```python
from build123d import *

# Parameters (mm, degrees)
SKETCH_1_R      = 100
SKETCH_1_R_2    = 10
EXTRUDE_1_DEPTH = 20
SKETCH_2_R      = 175
SKETCH_2_R_2    = 3
EXTRUDE_2_DEPTH = 10


with BuildPart() as part:
    # 草圖1 → 填料-伸長1 (new body)
    with BuildSketch(Plane(origin=(0, 0, 0), x_dir=(1, 0, 0), z_dir=(0, 1, 0))):
        with Locations(Location((0, 0, 0), (0, 0, 270))):
            Circle(SKETCH_1_R)
        with Locations(Location((0, 72.5, 0), (0, 0, 270))):
            Circle(SKETCH_1_R_2, mode=Mode.SUBTRACT)
        with Locations(Location((62.786841774, -36.25, 0), (0, 0, 270))):
            Circle(SKETCH_1_R_2, mode=Mode.SUBTRACT)
        with Locations(Location((-62.786841774, -36.25, 0), (0, 0, 270))):
            Circle(SKETCH_1_R_2, mode=Mode.SUBTRACT)
    extrude(amount=EXTRUDE_1_DEPTH)

    # 草圖2 → 填料-伸長2 (add)
    with BuildSketch(Plane.XZ):
        with Locations(Location((0, 0, 0), (0, 0, 270))):
            Circle(SKETCH_2_R)
        with Locations(Location((-150, 0, 0), (0, 0, 270))):
            Circle(SKETCH_2_R_2, mode=Mode.SUBTRACT)
        with Locations(Location((150, 0, 0), (0, 0, 270))):
            Circle(SKETCH_2_R_2, mode=Mode.SUBTRACT)
    extrude(amount=EXTRUDE_2_DEPTH)


solid = part.part
```
Input: part model. Units: mm. Frame: model coordinates. A direction names the side the tool comes from. Coordinates: 2 decimals unless noted, no trailing zeros. Write each loop counter-clockwise with the first axis right and the second up, starting at its lowest first coordinate (ties: lowest second). Pieces come first, ordered by that corner, then holes. Notation, with made-up numbers: M 63,28.25 L 85,28.25 A24 ccw 85,60.25 Z; hole C 61,20.25 d4. An arc over 180 degrees is marked long. Use one line per item in the form item = value.
Q1. Section D-D (z = 36). Return loops of the section in (x, y).
Answer below:
outline = M -171.26,-10 L 171.26,-10 L 171.26,0 L 93.3,0 L 93.3,20 L 72.78,20 L 72.78,0 L 52.79,0 L 52.79,20 L -52.79,20 L -52.79,0 L -72.78,0 L -72.78,20 L -93.3,20 L -93.3,0 L -171.26,0 Z
Q2. Draft query along Z for faces 1 (the face through (173.51, -4.93, 22.78)), 2 (the face through (-52.87, 9.86, 34.95)), 3 (the face through (2, -10, 2)). Return one class per face: released by +Z, released by -Z, zero draft, split by the parting line, or undercut.
Answer below:
face_1 = split by the parting line
face_2 = undercut
face_3 = zero draft
Q3. Material intervals for probe 1 along X at (y, z) = (-3.5, 0); probe 2 along X at (y, z) = (15.75, 36.25); probe 3 along Y at (x, z) = (12, -156), sorted ascending. Write a range as from..to.
Answer below:
probe_1 = -175..-153, -147..147, 153..175
probe_2 = -93.2..-72.79, -52.79..52.79, 72.79..93.2
probe_3 = -10..0
Q4. Section A-A (x = -20). Return loops of the section in (y, z).
Answer below:
outline = M -10,-173.85 L 0,-173.85 L 0,-97.98 L 20,-97.98 L 20,97.98 L 0,97.98 L 0,173.85 L -10,173.85 Z
Q5. Section B-B (z = -72.5). Return loops of the section in (x, y), plus the area to 3 significant figures.
Answer below:
outline = M -159.28,-10 L 159.28,-10 L 159.28,0 L 68.87,0 L 68.87,20 L 10,20 L 10,0 L -10,0 L -10,20 L -68.87,20 L -68.87,0 L -159.28,0 Z
area = 5,540 mm²
Q6. Set-up query: faces 4 (the face through (1, 20, -1)), 5 (the face through (63, 0, 36)). Return all of +Z, -Z, +X, -X, +Y, -Y with unobstructed straight access to the full face (end or side cutting, diameter ignored); none if empty.
Answer below:
face_4 = +Z, -Z, +X, -X, +Y
face_5 = +Y
Q7. First-contact query: pin 1 (2 mm diameter, centred on x = -51.5, y = 16.5, fed in from +Z); pin 2 (4 mm diameter, centred on x = 2, y = 3.5, fed in from -Z); pin 3 (10 mm diameter, centred on x = 0, z = -76, fed in from +Y). Flat tips, straight axial feed; report the tip coordinate or a pass-through.
Answer below:
pin_1 = 86.31
pin_2 = -100
pin_3 = 0
Q8. Section C-C (y = 8.5). Return loops of the section in (x, z), plus the area to 3 significant figures.
Answer below:
outline = C 0,0 d200; hole C -62.79,36.25 d20; hole C 0,-72.5 d20; hole C 62.79,36.25 d20
area = 30,500 mm²
